from build123d import *

# Parameters (mm, degrees)
DODANIE_WYCI_GNI_CIE1_DEPTH = 18
SKORUPA1_START              = 2
SKORUPA1_DEPTH              = 14
DODANIE_WYCI_GNI_CIE2_DEPTH = 18
WYTNIJ_WYCI_GNI_CIE1_REACH  = 32.228
WYTNIJ_WYCI_GNI_CIE2_REACH  = 32.228


# Read off the part's stored shape, not the designer's step: Skorupa1
with BuildPart() as part:
    # Szkic1 → Dodanie-wyciągnięcie1 (new body)
    with BuildSketch(Plane(origin=(0, 0, 0), x_dir=(1, 0, 0), z_dir=(0, 1, 0))):
        with BuildLine():
            Line((-15.171572875, 0), (0, 0))
            Line((0, 0), (0, 15.171572875))
            ThreePointArc((0, 15.171572875), (-1, 16.903623683), (-3, 16.903623683))
            Line((-3, 16.903623683), (-3, 3))
            Line((-3, 3), (-16.903623683, 3))
            ThreePointArc((-16.903623683, 3), (-16.903623683, 1), (-15.171572875, 0))
        make_face()
        with BuildLine():
            ThreePointArc((-16.585786438, 3.414213562), (-16.758279556, 3.217522858), (-16.903623683, 3))
            Line((-16.903623683, 3), (-3, 3))
            Line((-3, 3), (-3, 16.903623683))
            ThreePointArc((-3, 16.903623683), (-3.217522858, 16.758279556), (-3.414213562, 16.585786438))
            Line((-3.414213562, 16.585786438), (-16.585786438, 3.414213562))
        make_face()
    extrude(amount=DODANIE_WYCI_GNI_CIE1_DEPTH)

    # Skorupa1 outline → Skorupa1 (cut)
    with BuildSketch(Plane(origin=(0, 0, 0), x_dir=(1, 0, 0), z_dir=(0, 1, 0)).offset(SKORUPA1_START)):
        with BuildLine():
            Line((-3, 3), (-3, 15.171572875))
            Line((-3, 15.171572875), (0, 15.171572875))
            ThreePointArc((0, 15.171572875), (-1.234633135, 17.01933194), (-3.414213562, 16.585786438))
            Line((-3.414213562, 16.585786438), (-16.585786438, 3.414213562))
            ThreePointArc((-16.585786438, 3.414213562), (-17.01933194, 1.234633135), (-15.171572875, 0))
            Line((-15.171572875, 0), (-15.171572875, 3))
            Line((-15.171572875, 3), (-3, 3))
        make_face()
    extrude(amount=SKORUPA1_DEPTH, mode=Mode.SUBTRACT)

    # Szkic1<3> → Dodanie-wyciągnięcie2 (add)
    with BuildSketch(Plane(origin=(0, 0, 0), x_dir=(1, 0, 0), z_dir=(0, 1, 0))):
        with BuildLine():
            Line((-15.171572875, 0), (0, 0))
            Line((0, 0), (0, 15.171572875))
            ThreePointArc((0, 15.171572875), (-1, 16.903623683), (-3, 16.903623683))
            Line((-3, 16.903623683), (-3, 3))
            Line((-3, 3), (-16.903623683, 3))
            ThreePointArc((-16.903623683, 3), (-16.903623683, 1), (-15.171572875, 0))
        make_face()
    extrude(amount=DODANIE_WYCI_GNI_CIE2_DEPTH)

    # Szkic3 → Wytnij-wyciągnięcie1 (cut, up to next)
    with BuildSketch(Plane.XY, mode=Mode.PRIVATE) as wytnij_wyci_gni_cie1_sk1:
        with BuildLine():
            Line((-8.951811841, 7.5), (-10.951811841, 7.5))
            ThreePointArc((-10.951811841, 7.5), (-12.451811841, 9), (-10.951811841, 10.5))
            Line((-10.951811841, 10.5), (-8.951811841, 10.5))
            ThreePointArc((-8.951811841, 10.5), (-7.451811841, 9), (-8.951811841, 7.5))
        make_face()
    wytnij_wyci_gni_cie1_tool1 = extrude(wytnij_wyci_gni_cie1_sk1.sketch, amount=-WYTNIJ_WYCI_GNI_CIE1_REACH, mode=Mode.PRIVATE) & part.part
    add(wytnij_wyci_gni_cie1_tool1.solids().sort_by_distance((-9.951812, 9, 0))[0], mode=Mode.SUBTRACT)

    # Szkic4 → Wytnij-wyciągnięcie2 (cut, up to next)
    with BuildSketch(Plane(origin=(0, 0, 0), x_dir=(0, 0, -1), z_dir=(1, 0, 0)), mode=Mode.PRIVATE) as wytnij_wyci_gni_cie2_sk1:
        with BuildLine():
            Line((10.951811841, 7.5), (8.951811841, 7.5))
            ThreePointArc((8.951811841, 7.5), (7.451811841, 9), (8.951811841, 10.5))
            Line((8.951811841, 10.5), (10.951811841, 10.5))
            ThreePointArc((10.951811841, 10.5), (12.451811841, 9), (10.951811841, 7.5))
        make_face()
    wytnij_wyci_gni_cie2_tool1 = extrude(wytnij_wyci_gni_cie2_sk1.sketch, amount=-WYTNIJ_WYCI_GNI_CIE2_REACH, mode=Mode.PRIVATE) & part.part
    add(wytnij_wyci_gni_cie2_tool1.solids().sort_by_distance((0, 9, -9.951812))[0], mode=Mode.SUBTRACT)


solid = part.part
Input: part model. Units: mm. Frame: model coordinates. A direction names the side the tool comes from. Coordinates: 2 decimals unless noted, no trailing zeros. Loops run counter-clockwise (first coordinate to the right, second up) from the corner with the lowest first, then second, coordinate; pieces in that order, holes last. Notation, with made-up numbers: (36, 75) -> (81, 75) arc R26 cw to (81, 91) -> close; hole circle Ø4 at (38, 68.25). An arc over 180 degrees is marked (long way). Write each question's results on one line, items separated by ' | '. Start each with the question number.
Q1. Pin query (flat end, axial travel): pin 1 (2 mm diameter, centred on x = -12, z = -11.5, fed in from +Y); pin 2 (4 mm diameter, centred on y = 6.5, z = -13, fed in from -X); pin 3 (10 mm diameter, centred on x = -12.5, y = 2, fed in from -Z). Return the tip coordinate at first contact, or that it passes through.
Q2. Reachability of faces 1 (the flat face through (-10, 17, -10)), 2 (the flat face through (-1, 7.5, -10)), 3 (the flat face through (-10, 7, -3)), 4 (the flat face through (-6, 9, 0)), 5 (the cylindrical face through (-7.452, 9.033, -1.479)) from +Z, -Z, +X, -X, +Y, -Y: full face, straight path, thin tool, end or side. Return the list, or none.
Q3. Section B-B, the plane x = -9.75. Return the cut outline in (y, z).
Q4. Section C-C, the plane z = -10.5. Return the cut outline in (x, y).
Q5. Section D-D, the plane x = -13.5. Return the cut outline in (y, z).
Q6. Pull-direction query (Z, two-part tool) for faces 6 (the flat face through (0, 9, -6)), 7 (the flat face through (-10, 1, -10)), 8 (the cylindrical face through (-1.479, 8.967, -7.452)); classes: released by +Z, released by -Z, zero draft, split by the parting line, or undercut.
Q7. Ray query, line 1 (Y direction, x = -5, z = -10.5); line 2 (Z direction, x = -7, y = 9.75). Return the intervals inside material, ascending. Write a range as from..to.
Q8. Section A-A, the plane y = 9. Return the cut outline in (x, z).
Found:
1) pin 1: through | pin 2: x = -3 | pin 3: z = -12.5
2) face 1: -Z, -X, +Y, -Y | face 2: +X, -X | face 3: -Z, -X | face 4: +Z, +X, -X, +Y, -Y | face 5: +Z, -Z
3) outline: (0, -10.25) -> (2, -10.25) -> (2, -3) -> (7.5, -3) -> (7.5, 0) -> (0, 0) -> close; (10.5, -3) -> (16, -3) -> (16, -10.25) -> (18, -10.25) -> (18, 0) -> (10.5, 0) -> close
4) outline: (-9.5, 0) -> (0, 0) -> (0, 7.5) -> (-3, 7.5) -> (-3, 2) -> (-9.5, 2) -> close; (-9.5, 16) -> (-3, 16) -> (-3, 10.5) -> (0, 10.5) -> (0, 18) -> (-9.5, 18) -> close
5) outline: (0, -6.5) -> (2, -6.5) -> (2, -3) -> (16, -3) -> (16, -6.5) -> (18, -6.5) -> (18, 0) -> (0, 0) -> close
6) face 6: zero draft | face 7: released by -Z | face 8: undercut
7) line 1: 0..2, 16..18 | line 2: -3..0
8) outline: (-16.9, -3) -> (-12.45, -3) -> (-12.45, 0) -> (-15.17, 0) arc R2 ccw to start; (-7.45, -3) -> (-3, -3) -> (-3, -7.45) -> (0, -7.45) -> (0, 0) -> (-7.45, 0) -> close; (-3, -16.9) arc R2 ccw to (0, -15.17) -> (0, -12.45) -> (-3, -12.45) -> close
